Model file for the job. Use its own axes, mm. A direction names the side the tool comes from. Give positions to 0.01 mm unless a question says otherwise; leave off trailing zeros. Order: outer loops, then holes, each group sorted by start corner. A loop starts at its lowest first (then second) coordinate and runs counter-clockwise, first axis right, second up. Notation, with made-up numbers: (63.5, -1.5) - (122.5, -1.5) arc R23 cw to (122.5, 21.5) - close; hole circle Ø4 at (45, 22.5). An arc over 180 degrees is marked (long way). Use CSV: the item, a comma, the result in double quotes. Start each with the question number.
(1) Band-saw the part on B-B, the plane y = 60. Give the cut face in (x, z).
(2) Band-saw the part on A-A, the plane z = 18.5. Give the cut face in (x, y).
(3) Drop flat-ended pins along their axis: pin 1 Ø7.5 at (x, z) = (-52, -5) entering from +Y; pin 2 Ø3 at (x, y) = (53, 30.5) entering from +Z; pin 3 Ø0.5 at (x, y) = (0, 17.5) entering from -Z. Give the stop position or say it passes through.
(4) Band-saw the part on D-D, the plane z = -6. Give the cut face in (x, y), then the cut area to 3 significant figures.
(5) Band-saw the part on C-C, the plane x = 17.5. Give the cut face in (y, z), then the cut area to 3 significant figures.
(6) Probe L1, parallel to X at y = 60.5, z = 17.5; L2, parallel to X at y = 77, z = -8; L3, parallel to X at y = 26, z = -2. List the from-to ranges inside material, lowest first.
(7) Tool access for faces 1 (the flat face through (-1, 51, 10)), 2 (the flat face through (-72.43, 50.7, 20.14)), 3 (the cylindrical face through (17.17, 55.63, -0.004)): list every direction of +Z, -Z, +X, -X, +Y, -Y with a clear straight run to the whole face (end or side of a thin tool).
(8) Pull direction X, two halves, no side cores. Call faces 4 (the cylindrical face through (52.17, 55.63, -0.004)), 5 (the flat face through (77.5, 51, 3)), 6 (the flat face through (-0.4, 12.7, -15)): +X half, -X half, draft (parallel to the pull), parting line (faces both ways), or undercut.
from build123d import *

# Parameters (mm, degrees)
SKETCH1_W               = 155
SKETCH1_H               = 30
BOSS_EXTRUDE1_DEPTH     = 100
SKETCH2_R               = 15
CUT_EXTRUDE2_DEPTH      = 90
SKETCH4_W               = 155
SKETCH4_H               = 100
CUT_EXTRUDE3_DEPTH      = 5
BOSS_EXTRUDE2_DEPTH     = 155
SKETCH6_W               = 135
SKETCH6_H               = 20
CUT_EXTRUDE4_DEPTH      = 145
SKETCH7_W               = 5
SKETCH7_H               = 1
CUT_EXTRUDE6_DEPTH      = 1
CUT_EXTRUDE7_DEPTH      = 6
CUT_EXTRUDE7_DEPTH_BACK = 71
SKETCH8_W               = 1
SKETCH8_H               = 1
SKETCH9_W               = 5
SKETCH9_H               = 1
CUT_EXTRUDE8_DEPTH      = 1
CUT_EXTRUDE9_DEPTH      = 6
CUT_EXTRUDE9_DEPTH_BACK = 71
SKETCH10_W              = 1
SKETCH10_H              = 1


with BuildPart() as part:
    # Sketch1 → Boss-Extrude1 (new body)
    with BuildSketch(Plane(origin=(0, 0, 0), x_dir=(1, 0, 0), z_dir=(0, 1, 0))):
        Rectangle(SKETCH1_W, SKETCH1_H)
    extrude(amount=BOSS_EXTRUDE1_DEPTH)

    # Sketch2 → Cut-Extrude2 (cut)
    with BuildSketch(Plane(origin=(0, 100, 0), x_dir=(1, 0, 0), z_dir=(0, 1, 0))):
        with Locations((-52.5, 15)):
            Circle(SKETCH2_R)
        with Locations((-17.5, 15)):
            Circle(SKETCH2_R)
        with Locations((17.5, 15)):
            Circle(SKETCH2_R)
        with Locations((52.5, 15)):
            Circle(SKETCH2_R)
    extrude(amount=-CUT_EXTRUDE2_DEPTH, mode=Mode.SUBTRACT)

    # Sketch4 → Cut-Extrude3 (cut)
    with BuildSketch(Plane.XY.offset(15)):
        with Locations((0, 50)):
            Rectangle(SKETCH4_W, SKETCH4_H)
    extrude(amount=-CUT_EXTRUDE3_DEPTH, mode=Mode.SUBTRACT)

    # Sketch5 → Boss-Extrude2 (add)
    with BuildSketch(Plane(origin=(77.5, 0, 0), x_dir=(0, 0, -1), z_dir=(1, 0, 0))):
        Polygon((-10, 100), (-30, 100), (-10, 0), align=None)
    extrude(amount=-BOSS_EXTRUDE2_DEPTH)

    # Sketch6 → Cut-Extrude4 (cut)
    with BuildSketch(Plane(origin=(0, 100, 0), x_dir=(1, 0, 0), z_dir=(0, 1, 0))):
        with Locations((0, -20)):
            Rectangle(SKETCH6_W, SKETCH6_H)
    extrude(amount=-CUT_EXTRUDE4_DEPTH, mode=Mode.SUBTRACT)

    # Sketch7 → Cut-Extrude6 (cut)
    with BuildSketch(Plane(origin=(0, 0, -15), x_dir=(-1, 0, 0), z_dir=(0, 0, -1))):
        with Locations((-35, 13.5)):
            Rectangle(SKETCH7_W, SKETCH7_H)
    extrude(amount=-CUT_EXTRUDE6_DEPTH, mode=Mode.SUBTRACT)

    # Sketch8 → Cut-Extrude7 (cut, two sides: drawn at the far end of the back side and taken through both)
    with BuildSketch(Plane(origin=(32.5, 0, 0), x_dir=(0, 0, -1), z_dir=(1, 0, 0)).offset(-CUT_EXTRUDE7_DEPTH_BACK)):
        with Locations((14.5, 13.5)):
            Rectangle(SKETCH8_W, SKETCH8_H)
    extrude(amount=CUT_EXTRUDE7_DEPTH + CUT_EXTRUDE7_DEPTH_BACK, mode=Mode.SUBTRACT)

    # Sketch9 → Cut-Extrude8 (cut)
    with BuildSketch(Plane(origin=(0, 0, -15), x_dir=(-1, 0, 0), z_dir=(0, 0, -1))):
        with Locations((-35, 17.5)):
            Rectangle(SKETCH9_W, SKETCH9_H)
    extrude(amount=-CUT_EXTRUDE8_DEPTH, mode=Mode.SUBTRACT)

    # Sketch10 → Cut-Extrude9 (cut, two sides: drawn at the far end of the back side and taken through both)
    with BuildSketch(Plane(origin=(32.5, 0, 0), x_dir=(0, 0, -1), z_dir=(1, 0, 0)).offset(-CUT_EXTRUDE9_DEPTH_BACK)):
        with Locations((14.5, 17.5)):
            Rectangle(SKETCH10_W, SKETCH10_H)
    extrude(amount=CUT_EXTRUDE9_DEPTH + CUT_EXTRUDE9_DEPTH_BACK, mode=Mode.SUBTRACT)


solid = part.part
Answer block:
1,outline,"(-77.5, -15) - (-67.5, -15) arc R15 cw to (-37.5, -15) - (-32.5, -15) arc R15 cw to (-2.5, -15) - (2.5, -15) arc R15 cw to (32.5, -15) - (37.5, -15) arc R15 cw to (67.5, -15) - (77.5, -15) - (77.5, 22) - (67.5, 22) - (67.5, 10) - (-67.5, 10) - (-67.5, 22) - (-77.5, 22) - close"
2,outline,"(-77.5, 42.5) - (-67.5, 42.5) - (-67.5, 100) - (-77.5, 100) - close; (67.5, 42.5) - (77.5, 42.5) - (77.5, 100) - (67.5, 100) - close"
3,pin 1,"stops at y = 10"
3,pin 2,"stops at z = 10"
3,pin 3,"stops at z = -14"
4,outline,"(-77.5, 0) - (77.5, 0) - (77.5, 100) - (64.5, 100) - (64.5, 10) - (40.5, 10) - (40.5, 100) - (29.5, 100) - (29.5, 10) - (5.5, 10) - (5.5, 100) - (-5.5, 100) - (-5.5, 10) - (-29.5, 10) - (-29.5, 100) - (-40.5, 100) - (-40.5, 10) - (-64.5, 10) - (-64.5, 100) - (-77.5, 100) - close"
4,area,"6,860 mm2"
5,outline,"(0, -15) - (10, -15) - (10, 0) - (100, 0) - (100, 10) - (0, 10) - close"
5,area,"1,150 mm2"
6,L1,"x = -77.5 to -67.5, 67.5 to 77.5"
6,L2,"x = -77.5 to -65.77, -39.23 to -30.77, -4.23 to 4.23, 30.77 to 39.23, 65.77 to 77.5"
6,L3,"x = -77.5 to -59.98, -45.02 to -24.98, -10.02 to 10.02, 24.98 to 45.02, 59.98 to 77.5"
7,face 1,"+Z, +Y, -Y"
7,face 2,"+Z, +X, -X, -Y"
7,face 3,"-Z, +Y"
8,face 4,"undercut"
8,face 5,"+X half"
8,face 6,"draft"
